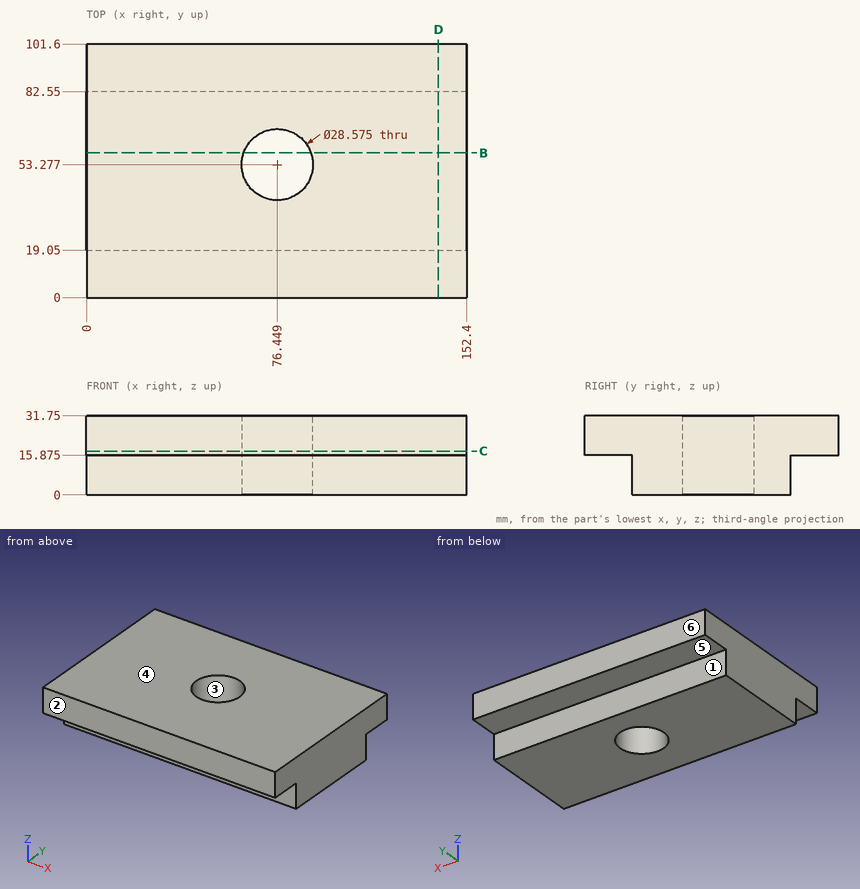
Geometry: see drawing. Coordinates: mm, zero at the bounding-box minimum. A direction names the side the tool comes from. Round coordinates to 2 decimals unless told otherwise and drop trailing zeros. Write each loop counter-clockwise with the first axis right and the second up, starting at its lowest first coordinate (ties: lowest second). Pieces come first, ordered by that corner, then holes. Notation, with made-up numbers: M -38.5,19 L -20.5,19 A10 cw -20.5,32 Z; hole C -7.75,76.25 d11. An arc over 180 degrees is marked long. Answer as a JSON object with one key per item and string values. Group by question number.
(1) Reachability of the marked faces 5 and 6 from +Z, -Z, +X, -X, +Y, -Y: full face, straight path, thin tool, end or side. Return the list, or none.
(2) Section query D-D on x = 141. Output: boundary loops of the cut face in (y, z) (3 decimals).
(3) Ray query, line 1 (Y direction, x = 131, z = 9); line 2 (Z direction, x = 65.5, y = 95) (3 decimals); line 3 (Y direction, x = 71.5, z = 9). Return the intervals inside material, ascending. Write a range as [from, to].
(4) Section query B-B on y = 58. Output: boundary loops of the cut face in (x, z).
(5) First-contact query: pin 1 (5 mm diameter, centred on x = 73, z = 7, fed in from -Y); pin 2 (17.5 mm diameter, centred on x = 73.5, z = 6, fed in from +Y); pin 3 (9.5 mm diameter, centred on x = 99, y = 95, fed in from -Z) (3 decimals). Flat tips, straight axial feed; report the tip coordinate or a pass-through.
(6) Section query C-C on z = 17.5. Output: boundary loops of the cut face in (x, y) (1 decimal), then the cut area to 3 significant figures.
(7) Mould query, pull axis Y, two halves, no side actions, for the marked faces 1, 2, 3 and 4. Classes: +Y half, -Y half, draft (parallel to the pull), parting line (faces both ways), or undercut.
Computed values:
{
 "1": {"face 5": "-Z, +X, -X, +Y", "face 6": "+Z, -Z, +X, -X, +Y"},
 "2": {"outline": "M 0,15.875 L 19.05,15.875 L 19.05,0 L 82.55,0 L 82.55,15.875 L 101.6,15.875 L 101.6,31.75 L 0,31.75 Z"},
 "3": {"line 1": "[19.05, 82.55]", "line 2": "[15.875, 31.75]", "line 3": "[19.05, 39.87], [66.68, 82.55]"},
 "4": {"outline": "M 0,0 L 62.96,0 L 62.96,31.75 L 0,31.75 Z; M 89.93,0 L 152.4,0 L 152.4,31.75 L 89.93,31.75 Z"},
 "5": {"pin 1": "y = 19.05", "pin 2": "y = 82.55", "pin 3": "z = 15.875"},
 "6": {"outline": "M 0,0 L 152.4,0 L 152.4,101.6 L 0,101.6 Z; hole C 76.4,53.3 d28.6", "area": "14,800 mm^2"},
 "7": {"face 1": "+Y half", "face 2": "-Y half", "face 3": "undercut", "face 4": "draft"}
}
